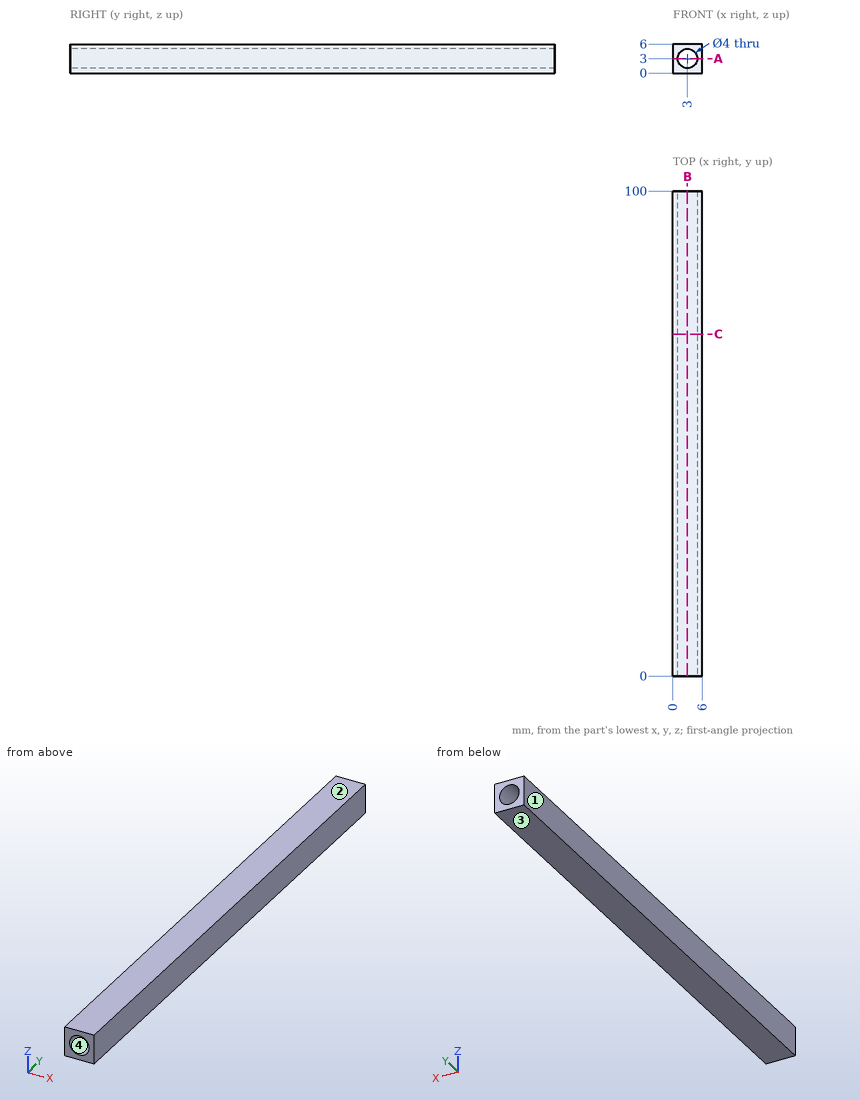
Study the drawing (mm; zero at the part's minimum x, y, z) and answer. Give positions to 0.01 mm unless a question says otherwise; leave off trailing zeros. Order: outer loops, then holes, each group sorted by start corner. A loop starts at its lowest first (then second) coordinate and runs counter-clockwise, first axis right, second up. Notation, with made-up numbers: M 16.25,-36 L 39.25,-36 A19 ccw 39.25,-12 Z; hole C 5,-31.75 d5. An arc over 180 degrees is marked long. Put each result on its own line as item: value. Start each with the question number.
Item 1: Find the intervals of material crossed by line 1 along Z through (x, y) = (3, 67); line 2 along X through (y, z) = (41.5, 4.35); line 3 along X through (y, z) = (50, 3.7), in increasing order.
Item 2: For a pull along Z with two mould halves and no side action, classify the marked faces 1, 2, 3 and 4 as +Z half, -Z half, draft (parallel to the pull), parting line (faces both ways), or undercut.
Item 3: The part is cut by section B-B, the plane x = 3. Determine the outline of the cut face in (y, z).
Item 4: A flat-ended cylindrical pin translates along its axis: P1, Ø3.5, axis at x = 3, z = 3, coming from the -Y side. Find the tip coordinate at first contact, or state that the pin passes through.
Item 5: The part is cut by section C-C, the plane y = 70.5. Determine the outline of the cut face in (x, z).
Item 6: The part is cut by section A-A, the plane z = 3. Determine the outline of the cut face in (x, y), and give its area (3 significant figures).
Answer key:
1. line 1: z = 0 to 1, 5 to 6
1. line 2: x = 0 to 1.52, 4.48 to 6
1. line 3: x = 0 to 1.13, 4.87 to 6
2. face 1: draft
2. face 2: +Z half
2. face 3: -Z half
2. face 4: undercut
3. outline: M 0,0 L 100,0 L 100,1 L 0,1 Z; M 0,5 L 100,5 L 100,6 L 0,6 Z
4. P1: passes through
5. outline: M 0,0 L 6,0 L 6,6 L 0,6 Z; hole C 3,3 d4
6. outline: M 0,0 L 1,0 L 1,100 L 0,100 Z; M 5,0 L 6,0 L 6,100 L 5,100 Z
6. area: 200 mm²
